Read the model definition and answer for the solid it produces. Units are mm, in the model's axes. A direction names the side the tool comes from. Round coordinates to 2 decimals unless told otherwise and drop trailing zeros. Order: outer loops, then holes, each group sorted by start corner. A loop starts at its lowest first (then second) coordinate and runs counter-clockwise, first axis right, second up. Notation, with made-up numbers: (13, 21.25) -> (29, 21.25) arc R10 cw to (29, 38.25) -> close; hole circle Ø9 at (72, 74.5). An arc over 180 degrees is marked (long way). Answer as a JSON object with one key per item and string values. Group by question number.
Item 1: Section A-A, the plane z = 2.85 is taken. Write down the section's boundary in (x, y).
Item 2: Section C-C, the plane x = -1 is taken. Write down the section's boundary in (y, z), plus the area to 3 significant figures.
Item 3: Section B-B, the plane y = 22.4 is taken. Write down the section's boundary in (x, z), plus the area to 3 significant figures.
Item 4: Section D-D, the plane y = 17.95 is taken. Write down the section's boundary in (x, z).
Item 5: The mould has two halves that part along Y. Classify faces 1 (the cylindrical face through (-7.21, 20.92, 5.7)), 2 (the cylindrical face through (8.274, 20.617, 2.465)), 3 (the cylindrical face through (7.685, 20.948, 2.465)): pulls with the +Y half, pulls with the -Y half, needs draft (parallel to the pull), parting line crosses it, or undercut.
Item 6: Given P1, Ø0.5, axis at x = -9, y = 18, coming from the +Z side; P2, Ø0.5, axis at x = -9.5, y = 18, coming from the -Z side; P3, Ø0.5, axis at y = 18, z = 2.5, coming from the -X side, each flat-ended and moving along its own axis, determine where each tip first touches the part or whether it passes through.
Item 7: Consider probe 1 along Y at (x, z) = (-3.75, 4.95); probe 2 along Y at (x, z) = (-10.25, 0.45); probe 3 along X at (y, z) = (22.2, 2). Determine where each line is inside the solid, lowest interval first. Write a range as from..to.
Item 8: For faces 4 (the flat face through (1, 22.673, 2)), 5 (the flat face through (-6.925, 19, 2)), 6 (the flat face through (-9, 18, 4.467)), determine the directions among +Z, -Z, +X, -X, +Y, -Y from which every point of the face is accessible in a straight line to the end or side of a thin tool.
from build123d import *

# Parameters (mm, degrees)
F1_DEPTH = 5
F2_DEPTH = 6
F3_W     = 3.613461
F3_H     = 3.543161
F4_DEPTH = 1
F5_R     = 1
F6_R     = 0.5


with BuildPart() as f1:
    # F0 (on Top) → F1 (new body)
    with BuildSketch(Plane.XY):
        with BuildLine():
            Line((8.470888, 23.242861), (-6.924916, 23.242861))
            Line((-6.924916, 23.242861), (-6.924916, 19.400692))
            Line((-6.924916, 19.400692), (6.014677, 19.400692))
            ThreePointArc((6.014677, 19.400692), (8.294767, 20.649267), (8.470888, 23.242861))
        make_face()
        with BuildLine():
            Line((-6.086436, 20.126112), (-6.086436, 22.673488))
            Line((-6.086436, 22.673488), (7.95457, 22.673488))
            ThreePointArc((7.95457, 22.673488), (7.669569, 20.927019), (6.091618, 20.126112))
            Line((6.091618, 20.126112), (-6.086436, 20.126112))
        make_face(mode=Mode.SUBTRACT)
    extrude(amount=F1_DEPTH)

    # F0 (on Top) → F2 (join)
    with BuildSketch(Plane.XY):
        Polygon((-6.924916, 23.242861), (-11.529112, 23.242861), (-11.529112, 18.535126), (-6.924916, 18.535126), (-6.924916, 19.400692), align=None)
    extrude(amount=F2_DEPTH)

    # F3 (on face) → F4 (join)
    with BuildSketch(Plane.XZ.offset(-18.535126)):
        with Locations((-9.175593, 2.695312)):
            Rectangle(F3_W, F3_H)
    extrude(amount=F4_DEPTH)

    # F5
    f5_edges = [f1.edges().sort_by_distance(p)[0] for p in [
        (-11.529112, 20.888994, 6),
        (-6.924916, 20.888994, 6),
        (-11.529112, 20.888994, 0),
    ]]
    fillet(f5_edges, radius=F5_R)

    # F6
    f6_edges = [f1.edges().sort_by_distance(p)[0] for p in [
        (-10.982323, 18.035126, 4.466893),
        (-7.368862, 18.035126, 4.466893),
        (-10.982323, 18.035126, 0.923732),
        (-7.368862, 18.035126, 0.923732),
    ]]
    fillet(f6_edges, radius=F6_R)


solid = f1.part
Values found:
{
 "1": {"outline": "(-11.53, 18.54) -> (-10.98, 18.54) -> (-10.98, 17.54) -> (-7.37, 17.54) -> (-7.37, 18.54) -> (-6.92, 18.54) -> (-6.92, 19.4) -> (6.01, 19.4) arc R2.71 ccw to (8.47, 23.24) -> (-11.53, 23.24) -> close; hole (-6.09, 20.13) -> (6.09, 20.13) arc R1.95 ccw to (7.95, 22.67) -> (-6.09, 22.67) -> close"},
 "2": {"outline": "(19.4, 0) -> (20.13, 0) -> (20.13, 5) -> (19.4, 5) -> close; (22.67, 0) -> (23.24, 0) -> (23.24, 5) -> (22.67, 5) -> close", "area": "6.47 mm2"},
 "3": {"outline": "(-11.53, 1) arc R1 ccw to (-10.53, 0) -> (-6.09, 0) -> (-6.09, 5) -> (-6.92, 5) arc R1 ccw to (-7.92, 6) -> (-10.53, 6) arc R1 ccw to (-11.53, 5) -> close; (8.02, 0) -> (8.7, 0) -> (8.7, 5) -> (8.02, 5) -> close", "area": "34.6 mm2"},
 "4": {"outline": "(-10.98, 1.42) arc R0.5 ccw to (-10.48, 0.92) -> (-7.87, 0.92) arc R0.5 ccw to (-7.37, 1.42) -> (-7.37, 3.97) arc R0.5 ccw to (-7.87, 4.47) -> (-10.48, 4.47) arc R0.5 ccw to (-10.98, 3.97) -> close"},
 "5": {"face 1": "needs draft", "face 2": "parting line crosses it", "face 3": "undercut"},
 "6": {"P1": "z = 4.47", "P2": "z = 0.92", "P3": "x = -10.98"},
 "7": {"probe 1": "19.4..20.13, 22.67..23.24", "probe 2": "18.54..23.24", "probe 3": "-11.53..-6.09, 8.04..8.72"},
 "8": {"face 4": "+Z, -Z", "face 5": "+Z, -Z, +X, -Y", "face 6": "+Z, +X, -X, -Y"}
}
